from build123d import *

# Parameters (mm, degrees)
F0_R      = 7.213779
F1_DEPTH  = 10
F2_DEPTH  = 10
F3_R      = 19
F4_DEPTH  = 10
F7_DEPTH  = 2.5
F8_DEPTH  = 2.5
F9_R      = 20.252872
F10_DEPTH = 20.822358


with BuildPart() as f1:
    # F0 (on Top) → F1 (new body)
    with BuildSketch(Plane.XY):
        Circle(F0_R)
        with BuildLine():
            ThreePointArc((2.448212, 4.359617), (4.315151, 2.525761), (5, 0))
            ThreePointArc((5, 0), (4.315151, -2.525761), (2.448212, -4.359617))
            ThreePointArc((2.448212, -4.359617), (-5, 0), (2.448212, 4.359617))
        make_face(mode=Mode.SUBTRACT)
    extrude(amount=F1_DEPTH)

    # F0 (on Top) → F2 (join)
    with BuildSketch(Plane.XY):
        with BuildLine():
            ThreePointArc((2.448212, -4.359617), (4.315151, -2.525761), (5, 0))
            ThreePointArc((5, 0), (4.315151, 2.525761), (2.448212, 4.359617))
            Line((2.448212, 4.359617), (2.448212, -4.359617))
        make_face()
    extrude(amount=F2_DEPTH)

    # F3 (on Top) → F4 (join)
    with BuildSketch(Plane.XY):
        Circle(F3_R)
    extrude(amount=-F4_DEPTH)

    # F5 (on Front) → F6 (revolve, cut)
    with BuildSketch(Plane.XZ):
        with BuildLine():
            Line((0, -30.822358), (0, -0.822358))
            ThreePointArc((0, -0.822358), (-15, -15.822358), (0, -30.822358))
        make_face()
    revolve(axis=Axis((0, 0, -15.822358), (0, 0, -1)), mode=Mode.SUBTRACT)

    # F5 (on Front) → F7 (join)
    with BuildSketch(Plane.XZ):
        with BuildLine():
            ThreePointArc((0, -30.822358), (10.606602, -26.42896), (15, -15.822358))
            ThreePointArc((15, -15.822358), (10.606602, -5.215757), (0, -0.822358))
            Line((0, -0.822358), (0, -30.822358))
        make_face()
        with BuildLine():
            Line((0, -30.822358), (0, -0.822358))
            ThreePointArc((0, -0.822358), (-15, -15.822358), (0, -30.822358))
        make_face()
    extrude(amount=F7_DEPTH)

    # F7_face (on face) → F8 (join)
    with BuildSketch(Plane(origin=(0, 0, -15.822358), x_dir=(1, 0, 0), z_dir=(0, 1, 0))):
        with BuildLine():
            ThreePointArc((-13.823898, -5.822358), (-8.296524, -12.496707), (0, -15))
            ThreePointArc((0, -15), (8.296524, -12.496707), (13.823898, -5.822358))
            ThreePointArc((13.823898, -5.822358), (0, 15), (-13.823898, -5.822358))
        make_face()
    extrude(amount=F8_DEPTH)

    # F9 (on face) → F10 (cut, through all)
    with BuildSketch(Plane(origin=(0, 0, -10), x_dir=(1, 0, 0), z_dir=(0, 0, -1))):
        Circle(F9_R)
    extrude(amount=F10_DEPTH, mode=Mode.SUBTRACT)


solid = f1.part
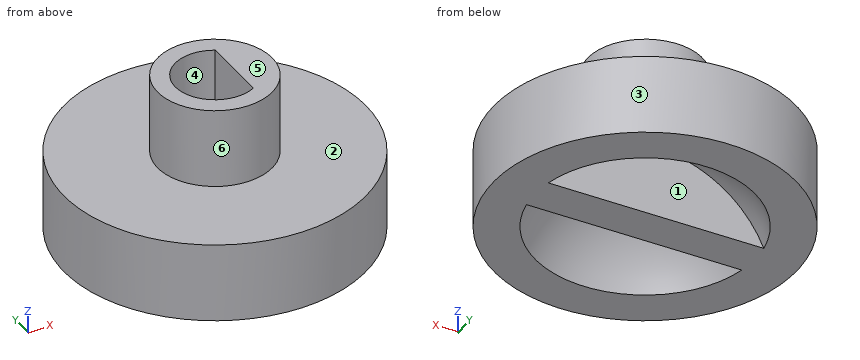
Read the model definition and answer for the solid it produces. Units are mm, in the model's axes. Face numbers are marked on the shaded views. A direction names the side the tool comes from. Round coordinates to 2 decimals unless told otherwise and drop trailing zeros. Write each loop counter-clockwise with the first axis right and the second up, starting at its lowest first coordinate (ties: lowest second). Pieces come first, ordered by that corner, then holes.
1. The part is cut by section C-C, the plane y = 0. Determine the outline of the cut face in (x, z), then the cut area to 3 significant figures.
2. The part is cut by section D-D, the plane z = 4.75. Determine the outline of the cut face in (x, y), then the cut area to 3 significant figures.
3. Given pin 1 Ø1 at (x, y) = (-8, -10.5) entering from +Z; pin 2 Ø12 at (x, z) = (-2, -0.5) entering from +Y; pin 3 Ø1.5 at (y, z) = (4.5, -7.5) entering from -X, each flat-ended and moving along its own axis, determine where each tip first touches the part or whether it passes through.
4. Straight lines are drawn through the part: L1, parallel to Y at x = 0, z = 7; L2, parallel to Y at x = 5.5, z = -9; L3, parallel to Y at x = 6.5, z = -5. For each, find the intervals that lie inside material, in ascending order.
5. The part is cut by section A-A, the plane z = -6.25. Determine the outline of the cut face in (x, y).
6. Determine the mould class of the marked faces 1, 2, 3 and 4 for opening direction Y: pulls with the +Y half, pulls with the -Y half, needs draft (parallel to the pull), parting line crosses it, or undercut.
7. The part is cut by section B-B, the plane x = 12. Determine the outline of the cut face in (y, z), then the cut area to 3 significant figures.
8. Which of the six approach directions +Z, -Z, +X, -X, +Y, -Y give full straight-line access (tool end or side, diameter ignored) to the marked faces 5 and 6?
Values:
1. outline: (-19, -10) - (19, -10) - (19, 0) - (7.21, 0) - (7.21, 10) - (2.45, 10) - (2.45, 0) - (-5, 0) - (-5, 10) - (-7.21, 10) - (-7.21, 0) - (-19, 0) - close
1. area: 450 mm2
2. outline: circle Ø14.43 at (0, 0); hole (2.45, -4.36) - (2.45, 4.36) arc R5 ccw (long way) to start
2. area: 101 mm2
3. pin 1: stops at z = 0
3. pin 2: stops at y = 19
3. pin 3: stops at x = -18.63
4. L1: y = -7.21 to -5, 5 to 7.21
4. L2: y = -18.19 to -12.17, -2.5 to 2.5, 12.17 to 18.19
4. L3: y = -17.85 to -8.1, -2.5 to 2.5, 8.1 to 17.85
5. outline: circle Ø38 at (0, 0); hole (-11.27, -2.5) arc R11.55 ccw to (11.27, -2.5) - close; hole (-11.27, 2.5) - (11.27, 2.5) arc R11.55 ccw to start
6. face 1: undercut
6. face 2: needs draft
6. face 3: parting line crosses it
6. face 4: undercut
7. outline: (-14.73, -10) - (-6.86, -10) arc R9 cw to (-2.5, -7.18) - (-2.5, -10) - (2.5, -10) - (2.5, -7.18) arc R9 cw to (6.86, -10) - (14.73, -10) - (14.73, 0) - (-14.73, 0) - close
7. area: 280 mm2
8. face 5: +Z, +X, -X, +Y, -Y
8. face 6: +Z
